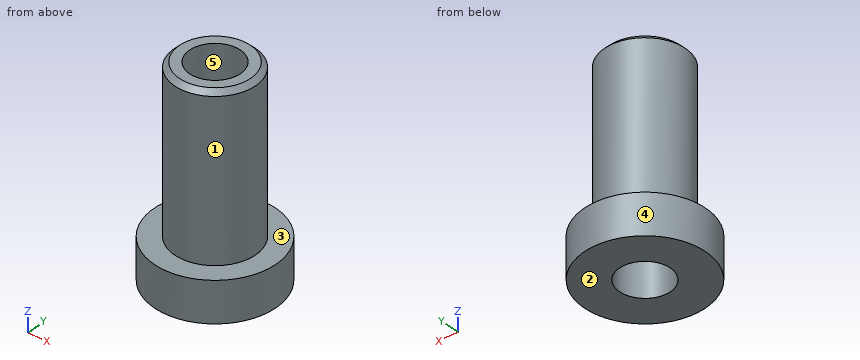
from build123d import *

# Parameters (mm, degrees)
SKETCH2_R          = 31.5
CUT_EXTRUDE1_DEPTH = 251


with BuildPart() as part:
    # Sketch1 → Revolve1 (revolve)
    with BuildSketch(Plane(origin=(0, 0, 0), x_dir=(1, 0, 0), z_dir=(0, 1, 0))):
        Polygon((0, 73.759969248), (75, 73.759969248), (75, 23.759969248), (50, 23.759969248), (50, -170.240030752), (44, -176.240030752), (0, -176.240030752), align=None)
    revolve(axis=Axis((0, 0, -73.759969248), (0, 0, 1)))

    # Sketch2 → Cut-Extrude1 (cut, through all)
    with BuildSketch(Plane.XY.offset(176.240030752)):
        Circle(SKETCH2_R)
    extrude(amount=-CUT_EXTRUDE1_DEPTH, mode=Mode.SUBTRACT)


solid = part.part
For this review, take the finished solid that the model builds, in its own axes (mm). Face numbers are marked on the shaded views. A direction names the side the tool comes from. Coordinates: 2 decimals unless noted, no trailing zeros. Order: outer loops, then holes, each group sorted by start corner. A loop starts at its lowest first (then second) coordinate and runs counter-clockwise, first axis right, second up. Notation, with made-up numbers: (74.5, 22) - (116.5, 22) arc R8 cw to (116.5, 29) - close; hole circle Ø8 at (46.5, 80.25). An arc over 180 degrees is marked (long way). Use one line per item in the form item = value.
Q1. Draft analysis for pull direction X (two halves, no side actions). For the marked faces 3, 4 and 5, state which applies: +X half, -X half, draft (parallel to the pull), parting line (faces both ways), or undercut.
Checked values:
face_3 = draft
face_4 = parting line
face_5 = undercut
Q2. For probe 1 along Y at (x, z) = (0, -14); probe 2 along Z at (x, y) = (14.5, 56); probe 3 along X at (y, z) = (-4, 27) (3 decimals), list the stretches that pass through material, from the lowest coordinate up. Write a range as from..to.
Checked values:
probe_1 = -50..-31.5, 31.5..50
probe_2 = -73.76..-23.76
probe_3 = -49.84..-31.245, 31.245..49.84
Q3. Consider section D-D (z = -28). Give the boundary of the cut face in (x, y).
Checked values:
outline = circle Ø150 at (0, 0); hole circle Ø63 at (0, 0)
Q4. For P1, Ø1.5, axis at y = -48.5, z = -44.5, coming from the -X side; P2, Ø4, axis at x = 43.5, y = 19.5, coming from the +Z side; P3, Ø8, axis at x = 19, y = 57.5, coming from the +Z side, all flat-tipped, find the tip position at first contact; note any pin that passes through.
Checked values:
P1 = -57.84
P2 = 174.57
P3 = -23.76
Q5. Consider section C-C (z = 62). Give the boundary of the cut face in (x, y).
Checked values:
outline = circle Ø100 at (0, 0); hole circle Ø63 at (0, 0)
Q6. For the marked faces 1 and 2, list the 3-axis set-ups (+Z, -Z, +X, -X, +Y, -Y) from which the entire face can be reached by the end or side of a thin tool; tool diameter is ignored.
Checked values:
face_1 = +Z
face_2 = -Z, +X, -X, +Y, -Y
Q7. Consider section A-A (y = 0). Give the boundary of the cut face in (x, z), then the cut area to 3 significant figures.
Checked values:
outline = (-75, -73.76) - (-31.5, -73.76) - (-31.5, 176.24) - (-44, 176.24) - (-50, 170.24) - (-50, -23.76) - (-75, -23.76) - close; (31.5, -73.76) - (75, -73.76) - (75, -23.76) - (50, -23.76) - (50, 170.24) - (44, 176.24) - (31.5, 176.24) - close
area = 11,700 mm2
